Drawing for the job (mm, zero at the part's lowest x, y, z). A direction names the side the tool comes from. Round coordinates to 2 decimals unless told otherwise and drop trailing zeros. Write each loop counter-clockwise with the first axis right and the second up, starting at its lowest first coordinate (ties: lowest second). Pieces come first, ordered by that corner, then holes. Notation, with made-up numbers: (47, 12.5) - (73, 12.5) arc R35 ccw to (73, 48.5) - close; hole circle Ø3 at (67.5, -27). An arc over 180 degrees is marked (long way). Answer in a Markdown table with one row per item.
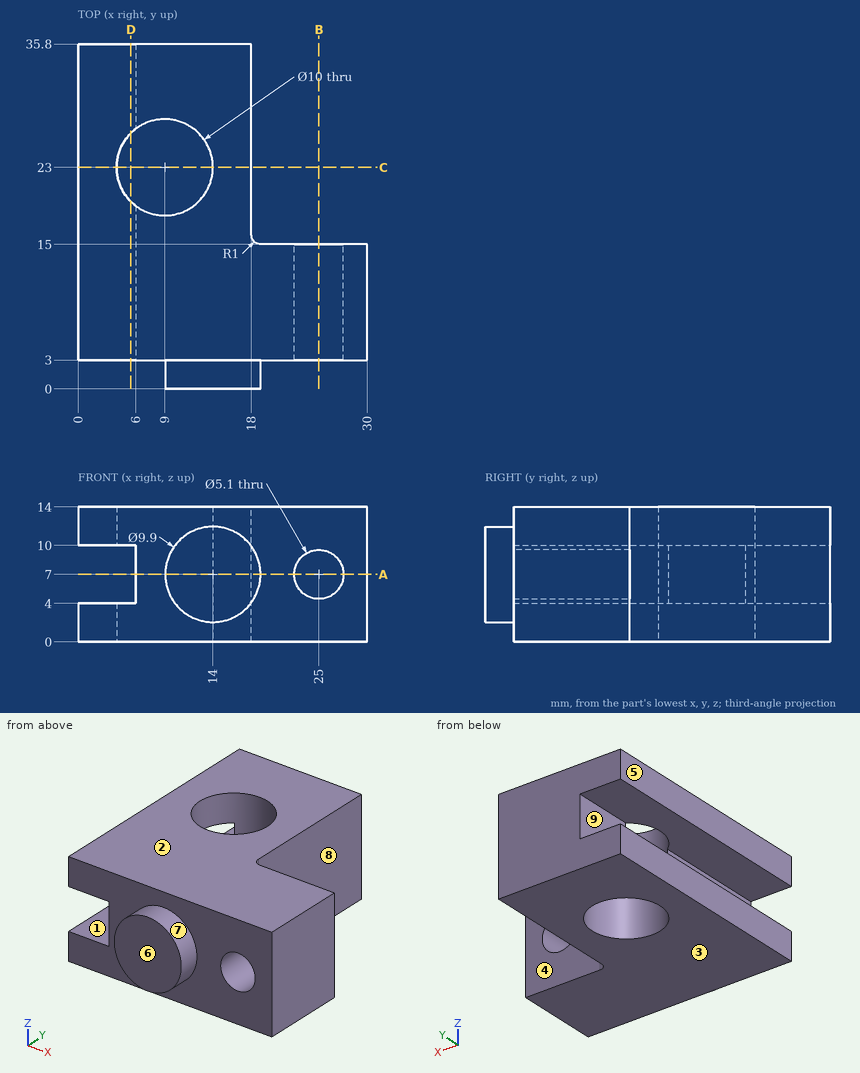
Q1. Pull direction Z, two halves, no side cores. Call the marked faces 1, 2, 3 and 4: released by +Z, released by -Z, zero draft, split by the parting line, or undercut.
Computed:
| item | result |
|---|---|
| face 1 | undercut |
| face 2 | released by +Z |
| face 3 | released by -Z |
| face 4 | zero draft |
Q2. Saw through at A-A on z = 7. List the corners of the cut face in (x, y), then the cut area to 3 significant figures.
Computed:
| item | result |
|---|---|
| outline | (6, 3) - (9.05, 3) - (9.05, 0) - (18.95, 0) - (18.95, 3) - (22.45, 3) - (22.45, 15) - (19, 15) arc R1 cw to (18, 16) - (18, 35.8) - (6, 35.8) - (6, 27) arc R5 cw (long way) to (6, 19) - close; (27.55, 3) - (30, 3) - (30, 15) - (27.55, 15) - close |
| area | 439 mm2 |
Q3. Saw through at D-D on x = 5.5. List the corners of the cut face in (y, z).
Computed:
| item | result |
|---|---|
| outline | (3, 0) - (19.43, 0) - (19.43, 4) - (3, 4) - close; (3, 10) - (19.43, 10) - (19.43, 14) - (3, 14) - close; (26.57, 0) - (35.8, 0) - (35.8, 4) - (26.57, 4) - close; (26.57, 10) - (35.8, 10) - (35.8, 14) - (26.57, 14) - close |
Q4. Flat gauge pins, fed straight in: pin 1 (1.8 mm diameter, centred on y = 13, z = 7.5, fed in from -X); pin 2 (16 mm diameter, centred on x = 9, y = 23, fed in from +Z); pin 3 (8 mm diameter, centred on x = 24, z = 12, fed in from -Y); pin 4 (8 mm diameter, centred on y = 23.5, z = 2.5, fed in from +X). Where does each tip first touch, or does it go through?
Computed:
| item | result |
|---|---|
| pin 1 | stops at x = 6 |
| pin 2 | stops at z = 14 |
| pin 3 | stops at y = 3 |
| pin 4 | stops at x = 18 |
Q5. Saw through at C-C on y = 23. List the corners of the cut face in (x, z).
Computed:
| item | result |
|---|---|
| outline | (0, 0) - (4, 0) - (4, 4) - (0, 4) - close; (0, 10) - (4, 10) - (4, 14) - (0, 14) - close; (14, 0) - (18, 0) - (18, 14) - (14, 14) - close |
Q6. 3-axis set-ups, long thin cutter, end or side, ignore diameter. For the marked faces 5, 6, 7, 8 and 9: which of +Z, -Z, +X, -X, +Y, -Y reach the whole face in a straight line?
Computed:
| item | result |
|---|---|
| face 5 | +Z, -Z, -X, +Y, -Y |
| face 6 | +Z, -Z, +X, -X, -Y |
| face 7 | -Y |
| face 8 | +Z, -Z, +X, +Y |
| face 9 | -X, +Y, -Y |
Q7. Saw through at B-B on x = 25. List the corners of the cut face in (y, z).
Computed:
| item | result |
|---|---|
| outline | (3, 0) - (15, 0) - (15, 4.45) - (3, 4.45) - close; (3, 9.55) - (15, 9.55) - (15, 14) - (3, 14) - close |
Q8. Drill centre lines: line 1 (Y direction, x = 9, z = 4); line 2 (X direction, y = 23, z = 9.5); line 3 (Y direction, x = 17.25, z = 13.25). Where is each one in solid material? Low to high.
Computed:
| item | result |
|---|---|
| line 1 | y = 3 to 18, 28 to 35.8 |
| line 2 | x = 14 to 18 |
| line 3 | y = 3 to 35.8 |
